Check sheet for the drawn part. Datum: minimum x, y, z corner. Units: mm. Give positions to 0.01 mm unless a question says otherwise; leave off trailing zeros. Order: outer loops, then holes, each group sorted by start corner. A loop starts at its lowest first (then second) coordinate and runs counter-clockwise, first axis right, second up. Notation, with made-up numbers: (-11, 77) -> (17, 77) arc R11 cw to (17, 87) -> close; hole circle Ø10 at (-32, 59.25). An arc over 180 degrees is marked (long way). Return JSON: item names as keys, results as strings. Group by question number.
(1) Cross-section at C-C on x = 25. Enter the section's corners in (y, z) (1 decimal).
(2) Thickness scan on line 1 along Y through (x, z) = (2.5, 31.5) (1 decimal); line 2 along Y through (x, z) = (38.5, 46) (1 decimal); line 3 along Z through (x, y) = (4, 73.5). Record the ranges inside material, lowest first.
(3) Release check for a two-part mould opening along Y. For the marked faces 1, 2, 3 and 4 record: pulls with the +Y half, pulls with the -Y half, needs draft (parallel to the pull), parting line crosses it, or undercut.
(4) Cross-section at A-A on z = 54. Enter the section's corners in (x, y), then the cut area to 3 significant figures.
(5) Cross-section at B-B on y = 72. Enter the section's corners in (x, z), then the cut area to 3 significant figures.
(6) Depth check by flat-ended pin: pin 1 Ø8 at (x, z) = (36, 31.5) entering from -Y. Enter the tip coordinate at first touch or a pass-through.
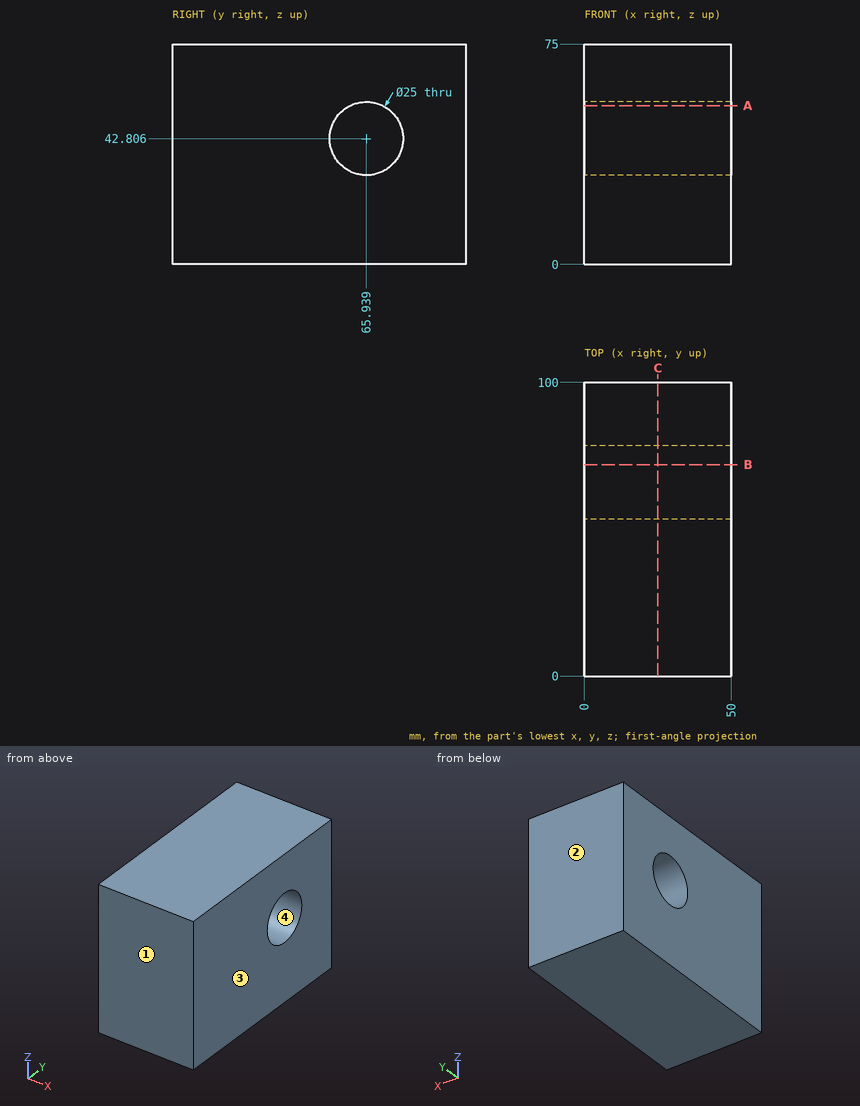
Verdict:
{
 "1": {"outline": "(0, 0) -> (100, 0) -> (100, 75) -> (0, 75) -> close; hole circle Ø25 at (65.9, 42.8)"},
 "2": {"line 1": "0 to 60.6, 71.3 to 100", "line 2": "0 to 53.9, 78 to 100", "line 3": "0 to 32.85, 52.76 to 75"},
 "3": {"face 1": "pulls with the -Y half", "face 2": "pulls with the +Y half", "face 3": "needs draft", "face 4": "undercut"},
 "4": {"outline": "(0, 0) -> (50, 0) -> (50, 60.38) -> (0, 60.38) -> close; (0, 71.5) -> (50, 71.5) -> (50, 100) -> (0, 100) -> close", "area": "4,440 mm²"},
 "5": {"outline": "(0, 0) -> (50, 0) -> (50, 31.87) -> (0, 31.87) -> close; (0, 53.74) -> (50, 53.74) -> (50, 75) -> (0, 75) -> close", "area": "2,660 mm²"},
 "6": {"pin 1": "y = 0"}
}
